from build123d import *
from build123d import SkipClean  # not in build123d's __all__

# Parameters (mm, degrees)
F0_R     = 34.0741
F0_R_2   = 30.1625
F1_DEPTH = 76.2
F2_R     = 34.0741
F2_R_2   = 30.1625
F3_DEPTH = 76.2
F4_R     = 34.0741
F4_R_2   = 27.6225
F5_DEPTH = 63.5
F6_R     = 30.1625
F7_DEPTH = 76.2
F8_R     = 27.6225
F9_DEPTH = 143.6


with BuildPart() as f1:
    # F0 (on Front) → F1 (new body, symmetric)
    with BuildSketch(Plane.XZ):
        Circle(F0_R)
        Circle(F0_R_2, mode=Mode.SUBTRACT)
    extrude(amount=F1_DEPTH, both=True)

    # F2 (on Top) → F3 (join)
    with BuildSketch(Plane.XY):
        Circle(F2_R)
        Circle(F2_R_2, mode=Mode.SUBTRACT)
    extrude(amount=F3_DEPTH)

    # F4 (on Front) → F5 (join, symmetric)
    with BuildSketch(Plane.XZ):
        Circle(F4_R)
        Circle(F4_R_2, mode=Mode.SUBTRACT)
    with SkipClean():  # cleaning this boolean's faces spoils the solid; the shape is the same uncleaned
        extrude(amount=F5_DEPTH, both=True)

    # F6 (on face) → F7 (cut, through all)
    with BuildSketch(Plane.XY.offset(76.2)):
        Circle(F6_R)
    extrude(amount=-F7_DEPTH, mode=Mode.SUBTRACT)

    # F8 (on Front) → F9 (cut, symmetric)
    with BuildSketch(Plane.XZ):
        Circle(F8_R)
    extrude(amount=F9_DEPTH, both=True, mode=Mode.SUBTRACT)


solid = f1.part
Build history of the part. All positions in model axes, mm. A direction names the side the tool comes from. Coordinates: 2 decimals unless noted, no trailing zeros. Order: outer loops, then holes, each group sorted by start corner. A loop starts at its lowest first (then second) coordinate and runs counter-clockwise, first axis right, second up. Notation, with made-up numbers: (12, 37) - (21, 37) arc R23 cw to (21, 72) - close; hole circle Ø9 at (71.25, -30). An arc over 180 degrees is marked (long way). Write item = value, one per line. Start each with the question number.
1) Two-plate mould, pull along X, no slides. Class faces 5 (the face through (12, -76.2, -28)), 6 (the face through (-7.387, -1.067, -33.264)), 7 (the face through (13.3, 63.5, -24.4)): pulls with the +X half, pulls with the -X half, needs draft (parallel to the pull), parting line crosses it, or undercut.
2) Saw through at D-D on y = 55. Write the cut outline in (x, z) (1 decimal), then the cut area to 3 significant figures.
3) Saw through at C-C on z = 62. Write the cut outline in (x, y) (1 decimal), then the cut area to 3 significant figures.
4) Flat gauge pins, fed straight in: pin 1 Ø6 at (y, z) = (-14, 41.5) entering from -X; pin 2 Ø1 at (x, z) = (19, 33.5) entering from +Y; pin 3 Ø8 at (y, z) = (-56.5, 13) entering from +X. Where does each tip first touch, or does it go through?
5) Saw through at A-A on x = 0. Write the cut outline in (y, z), then the cut area to 3 significant figures.
6) 3-axis set-ups, long thin cutter, end or side, ignore diameter. For faces 1 (the face through (-4.436, 33.784, 46.033)), 2 (the face through (12, 76.2, -28)), 3 (the face through (-30.133, 69.939, 1.326)), 4 (the face through (13.3, -63.5, -24.4)): which of +Z, -Z, +X, -X, +Y, -Y reach the whole face in a straight line?
7) Wall check: line 1 along X through (y, z) = (72, 0); line 2 along X through (y, z) = (15.5, 0). Give the ranges that are in metal, low to high. Write a range as from..to.
8) Saw through at B-B on z = 12. Write the cut outline in (x, y) (1 decimal), then the cut area to 3 significant figures.
From the geometry:
q1.face_5 = needs draft
q1.face_6 = parting line crosses it
q1.face_7 = undercut
q2.outline = circle Ø68.1 at (0, 0); hole circle Ø55.2 at (0, 0)
q2.area = 1,250 mm^2
q3.outline = circle Ø68.1 at (0, 0); hole circle Ø60.3 at (0, 0)
q3.area = 789 mm^2
q4.pin_1 = -32.25
q4.pin_2 = 28.61
q4.pin_3 = 32.86
q5.outline = (-76.2, -34.07) - (76.2, -34.07) - (76.2, -30.16) - (63.5, -30.16) - (63.5, -27.62) - (-63.5, -27.62) - (-63.5, -30.16) - (-76.2, -30.16) - close; (-76.2, 30.16) - (-63.5, 30.16) - (-63.5, 27.62) - (-30.16, 27.62) - (-30.16, 76.2) - (-34.07, 76.2) - (-34.07, 34.07) - (-76.2, 34.07) - close; (30.16, 27.62) - (63.5, 27.62) - (63.5, 30.16) - (76.2, 30.16) - (76.2, 34.07) - (34.07, 34.07) - (34.07, 76.2) - (30.16, 76.2) - close
q5.area = 1,780 mm^2
q6.face_1 = +Z
q6.face_2 = +Z, -Z, +X, -X, +Y
q6.face_3 = +Y
q6.face_4 = -Y
q7.line_1 = -34.07..-30.16, 30.16..34.07
q7.line_2 = -34.07..-27.62, 27.62..34.07
q8.outline = (-31.9, -76.2) - (-27.7, -76.2) - (-27.7, -63.5) - (-24.9, -63.5) - (-24.9, -17.1) arc R30.2 cw to (-24.9, 17.1) - (-24.9, 63.5) - (-27.7, 63.5) - (-27.7, 76.2) - (-31.9, 76.2) - (-31.9, 12) arc R34.1 ccw to (-31.9, -12) - close; (24.9, -63.5) - (27.7, -63.5) - (27.7, -76.2) - (31.9, -76.2) - (31.9, -12) arc R34.1 ccw to (31.9, 12) - (31.9, 76.2) - (27.7, 76.2) - (27.7, 63.5) - (24.9, 63.5) - (24.9, 17.1) arc R30.2 cw to (24.9, -17.1) - close
q8.area = 1,820 mm^2
